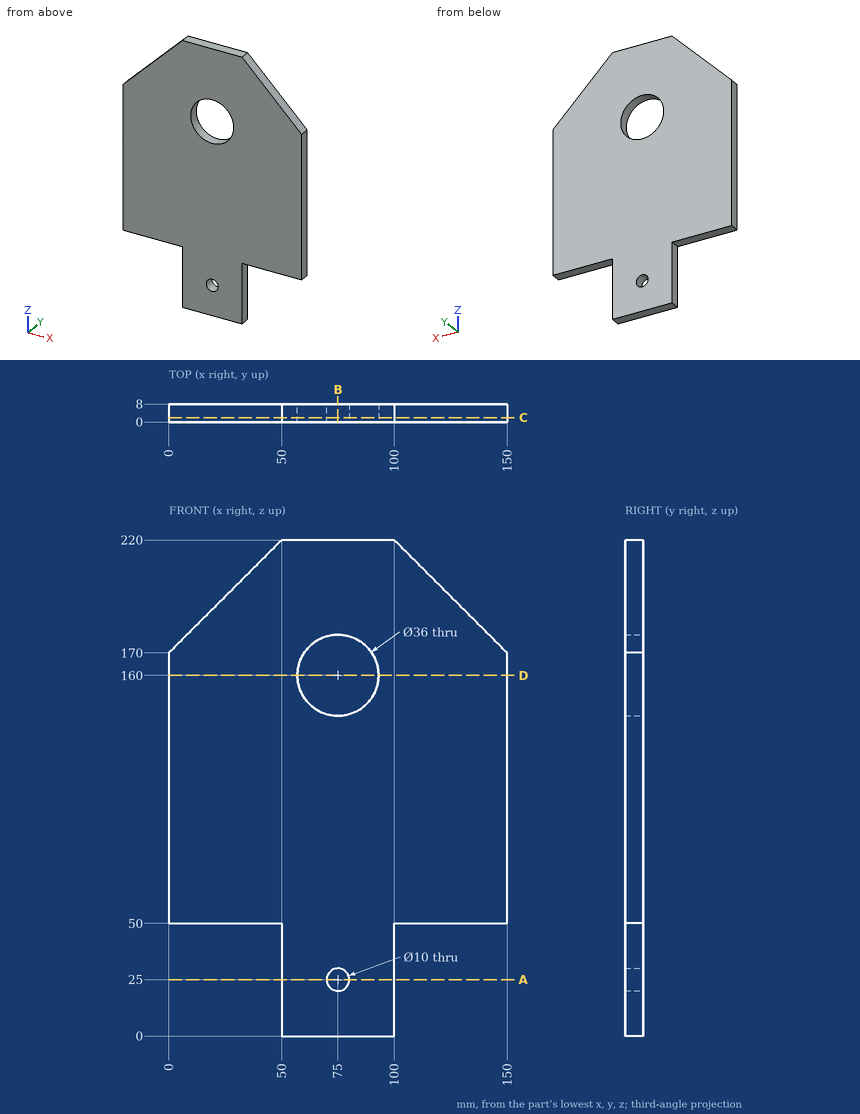
Print and shaded views of the part. All mm, measured from the part's lowest x, y and z. Round coordinates to 2 decimals unless told otherwise and drop trailing zeros. Write each loop counter-clockwise with the first axis right and the second up, starting at its lowest first coordinate (ties: lowest second). Pieces come first, ordered by that corner, then holes. Notation, with made-up numbers: M -31.5,79 L 4.5,79 A9 cw 4.5,92 Z; hole C 82.25,52.25 d10. An arc over 180 degrees is marked long. Use a Markdown table: item, result. Add a question column.
1. Flat gauge pins, fed straight in: P1, Ø2, axis at x = 123, y = 2.5, coming from the -Z side; P2, Ø2, axis at y = 6, z = 182, coming from the +X side; P3, Ø10, axis at x = 69, z = 97, coming from the -Y side; P4, Ø4, axis at y = 1, z = 181, coming from the -X side. Where does each tip first touch, or does it go through?
2. Slice it at B-B on x = 75. Give the cut face in (y, z).
3. Slice it at A-A on z = 25. Give the cut face in (x, y).
4. Slice it at D-D on z = 160. Give the cut face in (x, y), then the cut area to 3 significant figures.
5. Slice it at C-C on y = 2. Give the cut face in (x, z).
6. Drill centre lines: probe 1 along Z at (x, y) = (75, 3.75); probe 2 along X at (y, z) = (5.5, 160); probe 3 along X at (y, z) = (6, 26). Where is each one in solid material? Low to high.
Reply:
| question | item | result |
|---|---|---|
| 1 | P1 | stops at z = 50 |
| 1 | P2 | stops at x = 139 |
| 1 | P3 | stops at y = 0 |
| 1 | P4 | stops at x = 9 |
| 2 | outline | M 0,0 L 8,0 L 8,20 L 0,20 Z; M 0,30 L 8,30 L 8,142 L 0,142 Z; M 0,178 L 8,178 L 8,220 L 0,220 Z |
| 3 | outline | M 50,0 L 70,0 L 70,8 L 50,8 Z; M 80,0 L 100,0 L 100,8 L 80,8 Z |
| 4 | outline | M 0,0 L 57,0 L 57,8 L 0,8 Z; M 93,0 L 150,0 L 150,8 L 93,8 Z |
| 4 | area | 912 mm^2 |
| 5 | outline | M 0,50 L 50,50 L 50,0 L 100,0 L 100,50 L 150,50 L 150,170 L 100,220 L 50,220 L 0,170 Z; hole C 75,160 d36; hole C 75,25 d10 |
| 6 | probe 1 | z = 0 to 20, 30 to 142, 178 to 220 |
| 6 | probe 2 | x = 0 to 57, 93 to 150 |
| 6 | probe 3 | x = 50 to 70.1, 79.9 to 100 |
